Autodesk Fusion 360 part; units mm, degrees
sketch "Sketch1" plane through (0, 0, 0) normal (1, 0, 0) x (0, 0, -1)
  circle A0 centre (0, 0) radius 2.3995
  dimension "d1" = 4.799
extrude "Extrude1" add sketch "Sketch1" along normal blind 36
sketch "Sketch2" plane through (36, 0, 0) normal (1, 0, 0) x (0, 0, -1)
  circle A0 centre (0, 0) radius 2.3995
  line L0 (0.7, 2.3995) -> (-0.7, 2.3995)
  line L1 (-0.7, -2.3995) -> (0.7, -2.3995)
  line L2 (0.7, 2.3995) -> (-0.7, -2.3995) construction
  line L3 (-0.7, 2.3995) -> (0.7, -2.3995) construction
  line L4 (-2.3995, 0.7) -> (-2.3995, -0.7)
  line L5 (2.3995, -0.7) -> (2.3995, 0.7)
  line L6 (2.3995, 0.7) -> (-2.3995, -0.7) construction
  line L7 (-2.3995, 0.7) -> (2.3995, -0.7) construction
  line L8 (-0.7, 2.3995) -> (-0.7, 1)
  line L9 (-0.7, -1) -> (-0.7, -2.3995)
  line L10 (-2.3995, -0.7) -> (-1, -0.7)
  line L11 (1, -0.7) -> (2.3995, -0.7)
  line L12 (0.7, -2.3995) -> (0.7, -1)
  line L13 (0.7, 1) -> (0.7, 2.3995)
  line L14 (2.3995, 0.7) -> (1, 0.7)
  line L15 (-1, 0.7) -> (-2.3995, 0.7)
  arc A1 (-1, 0.7) -> (-0.7, 1) centre (-1, 1) ccw
  arc A2 (0.7, 1) -> (1, 0.7) centre (1, 1) ccw
  arc A3 (1, -0.7) -> (0.7, -1) centre (1, -1) ccw
  arc A4 (-0.7, -1) -> (-1, -0.7) centre (-1, -1) ccw
  dimension "d4" = 4.799
  dimension "d5" = 1.4
  dimension "d6" = 4.799
  dimension "d7" = 1.4
  dimension "d8" = 0.3
  dimension "d11" = 0.3
extrude "Extrude2" cut sketch "Sketch2" against normal blind 27 contours A0 L13 L14 A2 | A0 L11 L12 A3 | A0 L8 L15 A1 | A0 L9 L10 A4
sketch "Sketch4" plane through (0, 0, 0) normal (-1, 0, 0) x (0, 0, 1)
  circle A0 centre (0, 0) radius 2.3995
  circle A1 centre (0, 0) radius 2.3995
  arc A2 (2.2951, 0.7) -> (0.7, 2.2951) centre (0, 0) ccw
extrude "Extrude4" cut sketch "Sketch4" against normal blind 9
sketch "Sketch5" plane through (9, 0, 0) normal (-1, 0, 0) x (0, 0, 1)
  line L0 (-2.2951, -0.7) -> (-1, -0.7)
  arc A0 (-0.7, -1) -> (-1, -0.7) centre (-1, -1) ccw
  line L1 (-0.7, -1) -> (-0.7, -2.2951)
  arc A1 (-0.7, -2.2951) -> (0.7, -2.2951) centre (0, 0) ccw
  line L2 (0.7, -2.2951) -> (0.7, -1)
  arc A2 (1, -0.7) -> (0.7, -1) centre (1, -1) ccw
  line L3 (1, -0.7) -> (2.2951, -0.7)
  arc A3 (2.2951, -0.7) -> (2.2951, 0.7) centre (0, 0) ccw
  line L4 (2.2951, 0.7) -> (1, 0.7)
  arc A4 (0.7, 1) -> (1, 0.7) centre (1, 1) ccw
  line L5 (0.7, 1) -> (0.7, 2.2951)
  arc A5 (0.7, 2.2951) -> (-0.7, 2.2951) centre (0, 0) ccw
  line L6 (-0.7, 2.2951) -> (-0.7, 1)
  arc A6 (-1, 0.7) -> (-0.7, 1) centre (-1, 1) ccw
  line L7 (-1, 0.7) -> (-2.2951, 0.7)
  arc A7 (-2.2951, 0.7) -> (-2.2951, -0.7) centre (0, 0) ccw
  circle A8 centre (0, 0) radius 3
  dimension "d19" = 6
extrude "Extrude5" add sketch "Sketch5" along normal blind 11 contours L0 A0 L1 A1 L2 A2 L3 A3 L4 A4 L5 A5 L6 A6 L7 A7 | A8
sketch "Sketch6" plane through (-2, 0, 0) normal (-1, 0, 0) x (0, 0, 1)
  circle A0 centre (0, 0) radius 3
  line L0 (-1.25, 0) -> (-1.25, 1.3297)
  line L1 (-2.2951, 0.7) -> (-1, 0.7)
  line L2 (-1.25, 1.3297) -> (-1.25, -1.3297)
  arc A1 (-1.25, -1.3297) -> (-1.25, 1.3297) centre (0, 0) ccw
  point P0 (-0.7, -2.2951)
  dimension "d22" = 3.65
  dimension "d23" = 1.25
extrude "Extrude6" cut sketch "Sketch6" against normal blind 9 contours L0 L2 A1
fillet "Fillet3" radius 0.5 16 edges at (36, 2.3995, 0) (36, 0.7, -1.6476) (36, 0.7879, -0.7879) (36, 1.6476, -0.7) (36, 1.6476, 0.7) (36, 0.7879, 0.7879) (36, 0.7, 1.6476) (36, 0, 2.3995) (36, -0.7, 1.6476) (36, -0.7879, 0.7879) (36, -1.6476, 0.7) (36, -2.3995, 0) (36, -1.6476, -0.7) (36, -0.7879, -0.7879) (36, -0.7, -1.6476) (36, 0, -2.3995)
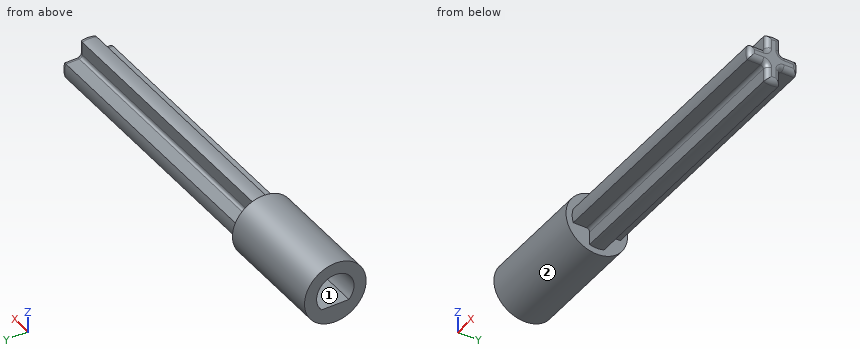
The model under review builds one solid part; all positions refer to its coordinate system, in mm. Face numbers are marked on the shaded views. Give positions to 0.01 mm unless a question says otherwise; leave off trailing zeros. Order: outer loops, then holes, each group sorted by start corner. A loop starts at its lowest first (then second) coordinate and runs counter-clockwise, first axis right, second up. Notation, with made-up numbers: (18, 44) -> (25, 44) arc R22 cw to (25, 64) -> close; hole circle Ø1 at (-26, -39). An arc over 180 degrees is marked (long way). Write item = value, one per line. Start each with the question number.
(1) Take a section at A-A (x = 32). Write out the cut boundary in (y, z), plus the area to 3 significant figures.
(2) For L1, parallel to Y at x = 1.75, z = 0 (3 decimals); L2, parallel to X at y = 2.2, z = 0.8; L3, parallel to Y at x = 29.5, z = 1.15, list the stretches that pass through material, from the lowest coordinate up. Write a range as from..to.
(3) Draft analysis for pull direction Z (two halves, no side actions). For the marked faces 1 and 2, state which applies: +Z half, -Z half, draft (parallel to the pull), parting line (faces both ways), or undercut.
(4) Take a section at B-B (x = 5). Write out the cut boundary in (y, z) (3 decimals).
(5) For pin 1 Ø0.6 at (x, y) = (19.5, -2) entering from +Z; pin 2 Ø0.6 at (x, y) = (22.5, 2) entering from -Z; pin 3 Ø1.5 at (x, y) = (16, -1) entering from +Z, all flat-tipped, find the tip position at first contact; note any pin that passes through.
Returned:
q1.outline = (-2.3, -0.7) -> (-1, -0.7) arc R0.3 cw to (-0.7, -1) -> (-0.7, -2.3) arc R2.4 ccw to (0.7, -2.3) -> (0.7, -1) arc R0.3 cw to (1, -0.7) -> (2.3, -0.7) arc R2.4 ccw to (2.3, 0.7) -> (1, 0.7) arc R0.3 cw to (0.7, 1) -> (0.7, 2.3) arc R2.4 ccw to (-0.7, 2.3) -> (-0.7, 1) arc R0.3 cw to (-1, 0.7) -> (-2.3, 0.7) arc R2.4 ccw to start
q1.area = 11.4 mm²
q2.L1 = -3..-1.825, 1.825..3
q2.L2 = -2..9
q2.L3 = -0.7..0.7
q3.face_1 = undercut
q3.face_2 = parting line
q4.outline = circle Ø6 at (0, 0); hole (-1.33, -1.25) -> (1.33, -1.25) arc R1.825 ccw (long way) to start
q5.pin_1 = 0.7
q5.pin_2 = -0.7
q5.pin_3 = 2.39
